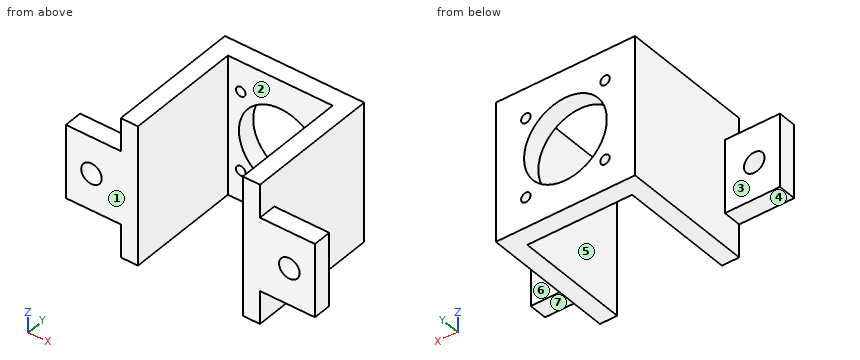
Autodesk Fusion 360 part; units mm, degrees
sketch "Sketch1" plane through (0, 0, 0) normal (0, 1, 0) x (1, 0, 0)
  line L0 (14, 14) -> (-14, 14)
  line L1 (-14, 14) -> (-14, -14)
  line L2 (-14, -14) -> (14, -14)
  line L3 (14, -14) -> (14, 14)
  line L4 (14, 14) -> (-14, -14) construction
  line L5 (-14, 14) -> (14, -14) construction
  line L6 (14, 14) -> (10.8, 14)
  line L7 (10.8, 14) -> (10.8, 10.8)
  circle A0 centre (10.8, 10.8) radius 1.3
  circle A1 centre (-10.8, 10.8) radius 1.3
  circle A2 centre (-10.8, -10.8) radius 1.3
  circle A3 centre (10.8, -10.8) radius 1.3
  line L8 (-19, 19) -> (19, 19)
  line L9 (19, 19) -> (19, -19)
  line L10 (19, -19) -> (-19, -19)
  line L11 (-19, -19) -> (-19, 19)
  line L12 (-19, 19) -> (19, -19) construction
  line L13 (19, 19) -> (-19, -19) construction
  circle A4 centre (0, 0) radius 11.3
  dimension "d1" = 28
  dimension "d2" = 28
  dimension "d3" = 3.2
  dimension "d4" = 3.2
  dimension "d5" = 2.6
  dimension "d7" = 360
  dimension "d8" = 38
  dimension "d9" = 38
  dimension "d10" = 22.6
extrude "Extrude1" add sketch "Sketch1" along normal blind 5 contours L0 L1 L2 L3 L6 | L8 L9 L10 L11
sketch "Sketch2" plane through (0, 0, 0) normal (0, 1, 0) x (1, 0, 0)
  circle A0 centre (10.8, 10.8) radius 1.3
  circle A1 centre (0, 0) radius 11.3
  circle A2 centre (10.8, -10.8) radius 1.3
  circle A3 centre (-10.8, -10.8) radius 1.3
  circle A4 centre (-10.8, 10.8) radius 1.3
  line L0 (19, -19) -> (-19, -19)
  line L1 (-19, -19) -> (-19, 19)
  line L2 (-19, 19) -> (19, 19)
  line L3 (19, 19) -> (19, -19)
  line L4 (14, 19) -> (14, -19)
  line L5 (-14, 19) -> (-14, -19)
  point P0 (-14, -14)
  point P1 (14, -14)
  point P2 (14, 14)
  point P3 (-14, 14)
extrude "Extrude2" add sketch "Sketch2" against normal blind 31.5 contours L0 L2 L3 L4 | L0 L1 L2 L5
extrude "Extrude3" cut 1 faces at (-14, -10.5, -6.3333) along direction (-1, 0, 0) blind 0.3
extrude "Extrude4" cut 1 faces at (14, -10.5, -6.3333) along direction (1, 0, 0) blind 0.3
sketch "Sketch3" plane through (-19, 0, 0) normal (-1, 0, 0) x (0, 0, 1)
  line L0 (19, -31.5) -> (19, 5)
  line L1 (19, 5) -> (-19, 5)
  line L2 (-19, 5) -> (-19, -31.5)
  line L3 (-19, -31.5) -> (19, -31.5)
  line L4 (0, -31.5) -> (-10, -31.5)
  line L5 (0, -31.5) -> (10, -31.5)
  line L6 (10, -31.5) -> (-10, -31.5)
  line L7 (-10, -31.5) -> (-10, -26.5)
  line L8 (-10, -26.5) -> (10, -26.5)
  line L9 (10, -26.5) -> (10, -31.5)
  dimension "d19" = 10
  dimension "d20" = 20
  dimension "d21" = 5
extrude "Extrude5" add sketch "Sketch3" along normal blind 15 contours L3 L4 L5 L6 L7 L8 L9
sketch "Sketch4" plane through (0, -26.5, 0) normal (0, 1, 0) x (-1, 0, 0)
  line L0 (19, 10) -> (19, -10)
  line L1 (19, -10) -> (34, -10)
  line L2 (34, -10) -> (34, 10)
  line L3 (34, 10) -> (19, 10)
  line L4 (34, 0) -> (27, 0)
  circle A0 centre (27, 0) radius 2.8
  dimension "d24" = 7
  dimension "d25" = 5.6
sketch "Sketch5" plane through (19, 0, 0) normal (1, 0, 0) x (0, 0, -1)
  line L0 (19, -31.5) -> (19, 5)
  line L1 (19, 5) -> (-19, 5)
  line L2 (-19, 5) -> (-19, -31.5)
  line L3 (-19, -31.5) -> (19, -31.5)
  line L4 (0, -31.5) -> (10, -31.5)
  line L5 (10, -31.5) -> (-10, -31.5)
  line L6 (-10, -31.5) -> (-10, -26.5)
  line L7 (-10, -26.5) -> (10, -26.5)
  line L8 (10, -26.5) -> (10, -31.5)
  dimension "d26" = 10
  dimension "d27" = 20
  dimension "d28" = 5
extrude "Extrude6" add sketch "Sketch5" along normal blind 15 contours L3 L4 L5 L6 L7 L8
sketch "Sketch6" plane through (0, -26.5, 0) normal (0, 1, 0) x (-1, 0, 0)
  line L0 (-19, -10) -> (-19, 10)
  line L1 (-19, 10) -> (-34, 10)
  line L2 (-34, 10) -> (-34, -10)
  line L3 (-34, -10) -> (-19, -10)
  line L4 (-34, 0) -> (-27, 0)
  circle A0 centre (-27, 0) radius 2.8
  dimension "d31" = 7
  dimension "d32" = 5.6
extrude "Extrude7" cut sketch "Sketch4" sketch "Sketch6" against normal blind 11 contours A0 of sketch 2 contours A0
Work out the finished part from the listing and answer in its coordinate system (mm). Face numbers are marked on the shaded views. A direction names the side the tool comes from. Give positions to 0.01 mm unless a question says otherwise; leave off trailing zeros. Write each loop counter-clockwise with the first axis right and the second up, starting at its lowest first coordinate (ties: lowest second). Pieces come first, ordered by that corner, then holes. Notation, with made-up numbers: (74.25, 81) -> (129.25, 81) arc R13 ccw to (129.25, 97) -> close; hole circle Ø5 at (46.25, 88.25). An arc over 180 degrees is marked (long way). Write each question's results on one line, items separated by ' | '.
1. A tool of negligible diameter and unlimited length cuts with its end or side. For the marked faces 3, 4, 5, 6 and 7, from which of +Z, -Z, +X, -X, +Y, -Y can it reach the whole face along a straight path? Write none if from no direction.
Data:
face 3: +Z, -Z, -X, +Y | face 4: -Z, -X, +Y, -Y | face 5: +Z, -Z, -Y | face 6: +Z, -Z, +X, +Y | face 7: -Z, +X, +Y, -Y
2. Find section A-A on y = -7. Determine the outline of the cut face in (x, z).
Data:
outline: (-19, -19) -> (-14.3, -19) -> (-14.3, 19) -> (-19, 19) -> close; (14.3, -19) -> (19, -19) -> (19, 19) -> (14.3, 19) -> close
3. Each of these flat-tipped pins is pushed along its axis until it touches: pin 1 Ø2.5 at (x, y) = (29.5, -28) entering from -Z; pin 2 Ø7.5 at (x, z) = (30, -4) entering from +Y; pin 3 Ø1 at (y, z) = (-9, 5) entering from +X. Where does it stop, or does it pass through?
Data:
pin 1: z = -10 | pin 2: y = -26.5 | pin 3: x = 19
4. Find section B-B on z = 0. Determine the outline of the cut face in (x, y).
Data:
outline: (-34, -31.5) -> (-29.8, -31.5) -> (-29.8, -26.5) -> (-34, -26.5) -> close; (-24.2, -31.5) -> (-14.3, -31.5) -> (-14.3, 0) -> (-11.3, 0) -> (-11.3, 5) -> (-19, 5) -> (-19, -26.5) -> (-24.2, -26.5) -> close; (11.3, 0) -> (14.3, 0) -> (14.3, -31.5) -> (24.2, -31.5) -> (24.2, -26.5) -> (19, -26.5) -> (19, 5) -> (11.3, 5) -> close; (29.8, -31.5) -> (34, -31.5) -> (34, -26.5) -> (29.8, -26.5) -> close
5. Find section C-C on x = 0. Determine the outline of the cut face in (y, z), and give its area (3 significant figures).
Data:
outline: (0, -19) -> (5, -19) -> (5, -11.3) -> (0, -11.3) -> close; (0, 11.3) -> (5, 11.3) -> (5, 19) -> (0, 19) -> close | area: 77.0 mm^2
6. Straight lines are drawn through the part: L1, parallel to X at y = -11.5, z = -1; L2, parallel to Z at x = 27, y = -29; L3, parallel to Z at x = 0, y = 1.65. For each, find the intervals that lie inside material, in ascending order.
Data:
L1: -19 to -14.3, 14.3 to 19 | L2: -10 to -2.8, 2.8 to 10 | L3: -19 to -11.3, 11.3 to 19
7. Find section D-D on y = 2. Determine the outline of the cut face in (x, z), and give its area (3 significant figures).
Data:
outline: (-19, -19) -> (19, -19) -> (19, 19) -> (-19, 19) -> close; hole circle Ø2.6 at (-10.8, -10.8); hole circle Ø2.6 at (-10.8, 10.8); hole circle Ø22.6 at (0, 0); hole circle Ø2.6 at (10.8, -10.8); hole circle Ø2.6 at (10.8, 10.8) | area: 1,020 mm^2
8. Determine the mould class of the marked faces 1 and 2 for opening direction X: +X half, -X half, draft (parallel to the pull), parting line (faces both ways), or undercut.
Data:
face 1: draft | face 2: undercut
